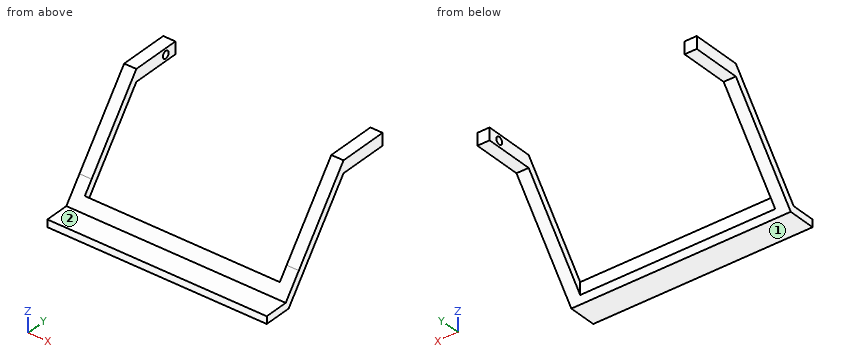
```python
from build123d import *

# Parameters (mm, degrees)
F0_W          = 25.7408986799
F0_H          = 6.35
F1_DEPTH      = 114.3
F2_W          = 101.6
F2_H          = 25.7408986799
F2_H_2        = 33.9491013201
F3_DEPTH      = 127
F5_R          = 1.905
F6_DEPTH      = 53.34
F6_DEPTH_BACK = 53.34


with BuildPart() as f1:
    # F0 (on Right) → F1 (new body)
    with BuildSketch(Plane.YZ):
        with Locations((-8.492361987, 0)):
            Rectangle(F0_W, F0_H)
        Polygon((-21.362811327, 3.175), (-50.8, -35.5794671973), (-50.8, -41.9294671973), (-21.362811327, -3.175), align=None)
        Polygon((-62.3238671319, -50.7507981185), (-59.429860403, -46.9407981185), (-71.9224512577, -46.9407981185), (-71.9224512577, -50.7507981185), align=None)
        Polygon((-50.8, -41.9294671973), (-50.8, -35.5794671973), (-59.429860403, -46.9407981185), (-57.5005225837, -46.9407981185), (-57.5005225837, -50.7507981185), align=None)
        Polygon((-57.5005225837, -46.9407981185), (-59.429860403, -46.9407981185), (-62.3238671319, -50.7507981185), (-57.5005225837, -50.7507981185), align=None)
    extrude(amount=F1_DEPTH)

    # F2 (on face) → F3 (cut)
    with BuildSketch(Plane.XY.offset(3.175)):
        with Locations((57.15, -8.492361987)):
            Rectangle(F2_W, F2_H)
        with Locations((57.15, -38.337361987)):
            Rectangle(F2_W, F2_H_2)
    extrude(amount=-F3_DEPTH, mode=Mode.SUBTRACT)

    # F5 (on offset) → F6 (cut, two sides)
    with BuildSketch(Plane(origin=(57.15, 0, 0), x_dir=(0, -1, 0), z_dir=(-1, 0, 0))) as f6_sk:
        with Locations((1.971912647, 0)):
            Circle(F5_R)
    extrude(amount=-F6_DEPTH, mode=Mode.SUBTRACT)
    extrude(f6_sk.sketch, amount=F6_DEPTH_BACK, mode=Mode.SUBTRACT)


solid = f1.part
```
Geometry: final body of the model. Coordinates: model frame, mm. Face numbers are marked on the shaded views. A direction names the side the tool comes from. Give positions to 0.01 mm unless a question says otherwise; leave off trailing zeros. Loops run counter-clockwise (first coordinate to the right, second up) from the corner with the lowest first, then second, coordinate; pieces in that order, holes last. Notation, with made-up numbers: (-13.5, 0) - (-2.5, 0) arc R18 cw to (-2.5, 10) - close; hole circle Ø8 at (64, 65). An arc over 180 degrees is marked (long way). Answer as CSV lines item,"result". Start each with the question number.
(1) Section query C-C (x = 74). Output: boundary loops of the cut face in (y, z).
(2) Section query A-A (y = -19). Output: boundary loops of the cut face in (x, z) (3 decimals).
(3) Pin query (flat end, axial travel): P1, Ø3, axis at x = 52, y = -54.5, coming from the -Z side; P2, Ø4, axis at x = 23, y = -53.5, coming from the +Z side; P3, Ø6, axis at x = 58, y = -67, coming from the +Z side. Return the tip coordinate at first contact, or that it passes through.
(4) Section query B-B (z = 0). Output: boundary loops of the cut face in (x, y), and give its area (3 significant figures).
(5) Ray query, line 1 along X through (y, z) = (-16.5, -2); line 2 along Y through (x, z) = (4.75, 0); line 3 along Z through (x, y) = (75, -67). Return the intervals inside material, ascending. Write a range as [from, to].
(6) Section query D-D (z = -25). Output: boundary loops of the cut face in (x, y).
(7) Reachability of the marked faces 1 and 2 from +Z, -Z, +X, -X, +Y, -Y: full face, straight path, thin tool, end or side. Return the list, or none.
Worked answers:
1,outline,"(-71.92, -50.75) - (-57.5, -50.75) - (-55.31, -47.87) - (-55.31, -41.52) - (-59.43, -46.94) - (-71.92, -46.94) - close"
2,outline,"(0, -3.175) - (6.35, -3.175) - (6.35, 3.175) - (0, 3.175) - close; (107.95, -3.175) - (114.3, -3.175) - (114.3, 3.175) - (107.95, 3.175) - close"
3,P1,"stops at z = -48.78"
3,P2,"stops at z = -41.52"
3,P3,"stops at z = -46.94"
4,outline,"(0, -23.77) - (6.35, -23.77) - (6.35, -3.88) - (3.81, -3.88) - (3.81, -0.07) - (6.35, -0.07) - (6.35, 4.38) - (0, 4.38) - close; (107.95, -23.77) - (114.3, -23.77) - (114.3, 4.38) - (107.95, 4.38) - (107.95, -0.07) - (110.49, -0.07) - (110.49, -3.88) - (107.95, -3.88) - close"
4,area,"338 mm^2"
5,line 1,"x = [0, 6.35], [107.95, 114.3]"
5,line 2,"y = [-23.77, -3.88], [-0.07, 4.38]"
5,line 3,"z = [-50.75, -46.94]"
6,outline,"(0, -42.76) - (6.35, -42.76) - (6.35, -37.94) - (0, -37.94) - close; (107.95, -42.76) - (114.3, -42.76) - (114.3, -37.94) - (107.95, -37.94) - close"
7,face 1,"-Z, +X, -X, +Y, -Y"
7,face 2,"+Z, +X, -X, -Y"
